The listing builds one solid part. Answer for the finished solid, in the listing's coordinates (mm). Round coordinates to 2 decimals unless told otherwise and drop trailing zeros. Write each loop counter-clockwise with the first axis right and the second up, starting at its lowest first coordinate (ties: lowest second). Pieces come first, ordered by that corner, then holes. Notation, with made-up numbers: (53, -28) - (93, -28) arc R25 ccw to (93, 1) - close; hole circle Ø3 at (4, 35). An arc over 180 degrees is marked (long way). Use a Markdown table: item, result. Add a question column.
1) Find the intervals of material crossed by probe 1 along X at (y, z) = (0.55, 0.5); probe 2 along X at (y, z) = (0.05, -0.5); probe 3 along Z at (x, y) = (21.5, 0.25), in increasing order. Write a range as from..to.
2) A cutting plane is placed at C-C (y = 0.5). Give the vertices of the cut face in (x, z), then the cut area to 3 significant figures.
3) A cutting plane is placed at A-A (z = -0.5). State how many separate pieces and enclosed holes the cut face has, then the cut area to 3 significant figures.
4) This flat-tipped pin is pushed along its axis until it touches: P1, Ø2.5, axis at x = 43.71, z = -0.5, coming from the -Y side. Where does it stop, or does it pass through?
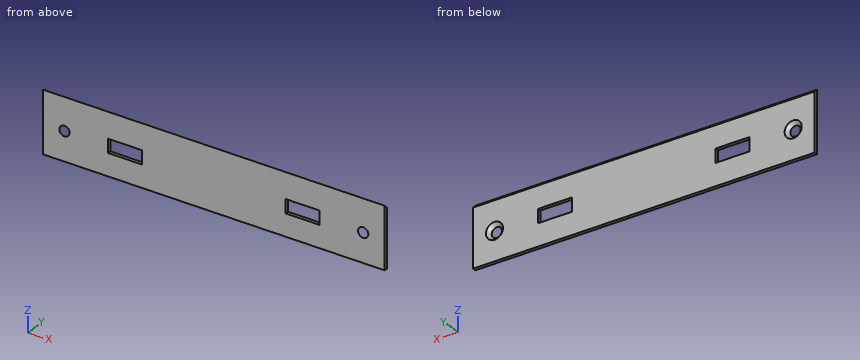
```python
from build123d import *

# Parameters (mm, degrees)
SKETCH_1_W          = 100
SKETCH_1_H          = 18
EXTRUDE_1_DEPTH     = 1
CHAMFER_1_SIZE      = 1
SKETCH_2_W          = 10
SKETCH_2_H          = 4
CUT_EXTRUDE_1_DEPTH = 1
SKETCH_3_R          = 1.5
CUT_EXTRUDE_2_DEPTH = 20
CHAMFER_2_SIZE      = 1


with BuildPart() as part:
    # Эскиз1 → Бобышка-Вытянуть1 (new body)
    with BuildSketch(Plane(origin=(0, 0, 0), x_dir=(1, 0, 0), z_dir=(0, 1, 0))):
        Rectangle(SKETCH_1_W, SKETCH_1_H)
    extrude(amount=EXTRUDE_1_DEPTH)

    # Фаска1
    chamfer_1_edges = [part.edges().sort_by_distance(p)[0] for p in [
        (0, 1, 9),
    ]]
    chamfer(chamfer_1_edges, length=CHAMFER_1_SIZE - 0.0001)  # a hair under: the kernel refuses the full size

    # Эскиз2 → Вырез-Вытянуть1 (cut)
    with BuildSketch(Plane(origin=(0, 1, 0), x_dir=(1, 0, 0), z_dir=(0, 1, 0))):
        with Locations((-26, 0.5)):
            Rectangle(SKETCH_2_W, SKETCH_2_H)
        with Locations((26, 0.5)):
            Rectangle(SKETCH_2_W, SKETCH_2_H)
    extrude(amount=-CUT_EXTRUDE_1_DEPTH, mode=Mode.SUBTRACT)

    # Эскиз3 → Вырез-Вытянуть2 (cut)
    with BuildSketch(Plane(origin=(0, 1, 0), x_dir=(1, 0, 0), z_dir=(0, 1, 0))):
        with Locations(Location((-43.709679881, 0.5, 0), (0, 0, 270))):
            Circle(SKETCH_3_R)
        with Locations(Location((43.709679881, 0.5, 0), (0, 0, 90))):
            Circle(SKETCH_3_R)
    extrude(amount=-CUT_EXTRUDE_2_DEPTH, mode=Mode.SUBTRACT)

    # Фаска2
    chamfer_2_edges = [part.edges().sort_by_distance(p)[0] for p in [
        (-43.709679881, 1, -2),
        (43.709679881, 1, 1),
    ]]
    chamfer(chamfer_2_edges, length=CHAMFER_2_SIZE - 0.0001)  # a hair under: the kernel refuses the full size


solid = part.part
```
Entries:
| question | item | result |
|---|---|---|
| 1 | probe 1 | x = -50..-45.5, -41.92..-31, -21..21, 31..41.92, 45.5..50 |
| 1 | probe 2 | x = -50..-45.26, -42.16..-31, -21..21, 31..42.16, 45.26..50 |
| 1 | probe 3 | z = -9..-2.5, 1.5..8.75 |
| 2 | outline | (-50, -9) - (50, -9) - (50, 8.5) - (-50, 8.5) - close; hole circle Ø4 at (-43.71, -0.5); hole (-31, -2.5) - (-21, -2.5) - (-21, 1.5) - (-31, 1.5) - close; hole (21, -2.5) - (31, -2.5) - (31, 1.5) - (21, 1.5) - close; hole circle Ø4 at (43.71, -0.5) |
| 2 | area | 1,640 mm² |
| 3 | separate pieces | 5 |
| 3 | enclosed holes | 0 |
| 3 | area | 72.0 mm² |
| 4 | P1 | passes through |
